from build123d import *

# Parameters (mm, degrees)
F0_W     = 125
F0_H     = 80
F0_W_2   = 121
F0_H_2   = 76
F1_DEPTH = 4
F2_W     = 121
F2_H     = 76
F3_DEPTH = 1
F4_W     = 30
F4_H     = 101.913806
F4_H_2   = 48.086194
F5_DEPTH = 10
F6_W     = 80
F6_H     = 30
F6_W_2   = 30
F6_H_2   = 10
F7_DEPTH = 5


with BuildPart() as f1:
    # F0 (on Front) → F1 (new body)
    with BuildSketch(Plane.XZ):
        Rectangle(F0_W, F0_H)
        Rectangle(F0_W_2, F0_H_2, mode=Mode.SUBTRACT)
        Rectangle(F0_W_2, F0_H_2)
    extrude(amount=F1_DEPTH)

    # F2 (on face) → F3 (cut)
    with BuildSketch(Plane.XZ.offset(4)):
        Rectangle(F2_W, F2_H)
    extrude(amount=-F3_DEPTH, mode=Mode.SUBTRACT)

    # F4 (on face) → F5 (join)
    with BuildSketch(Plane.XZ):
        with Locations((0, -88.956903)):
            Rectangle(F4_W, F4_H)
        with Locations((0, -13.956903)):
            Rectangle(F4_W, F4_H_2)
    extrude(amount=-F5_DEPTH)

    # F6 (on face) → F7 (join)
    with BuildSketch(Plane(origin=(0, 0, -139.913806), x_dir=(1, 0, 0), z_dir=(0, 0, -1))):
        with Locations((0, -5)):
            Rectangle(F6_W, F6_H)
        with Locations((0, -5)):
            Rectangle(F6_W_2, F6_H_2, mode=Mode.SUBTRACT)
    extrude(amount=-F7_DEPTH)


solid = f1.part
The listing builds one solid part. Answer for the finished solid, in the listing's coordinates (mm). A direction names the side the tool comes from. Give positions to 0.01 mm unless a question says otherwise; leave off trailing zeros. Write each loop counter-clockwise with the first axis right and the second up, starting at its lowest first coordinate (ties: lowest second). Pieces come first, ordered by that corner, then holes.
1) For a pull along Z with two mould halves and no side action, classify faces 1 (the face through (-1, 11, -134.914)), 2 (the face through (-1, 5, -139.914)), 3 (the face through (-1, 20, -137)) as pulls with the +Z half, pulls with the -Z half, needs draft (parallel to the pull), parting line crosses it, or undercut.
2) A tool of negligible diameter and unlimited length cuts with its end or side. For faces 4 (the face through (0, 10, -61)), 5 (the face through (0, -4, 39)), 6 (the face through (-1, -2, -40)), 7 (the face through (-1, -3, 1)), from which of +Z, -Z, +X, -X, +Y, -Y can it reach the whole face along a straight path? Write none if from no direction.
3) Find the intervals of material crossed by L1, parallel to Z at x = 28, y = -2.5; L2, parallel to X at y = 8.25, z = -58.5; L3, parallel to Z at x = -26, y = -5, in increasing order.
4) Section A-A (x = 32.5) is taken. Write down the section's boundary in (y, z).
5) Section D-D (y = 7.75) is taken. Write down the section's boundary in (x, z).
6) Section C-C (z = -18.5) is taken. Write down the section's boundary in (x, y), and give its area (3 significant figures).
7) Given P1, Ø4, axis at y = 6, z = -136.5, coming from the +X side; P2, Ø3, axis at y = 5.5, z = -86, coming from the -X side; P3, Ø24, axis at x = -30, z = 4.5, coming from the +Y side, each flat-ended and moving along its own axis, determine where each tip first touches the part or whether it passes through.
8) Section B-B (x = -12.5) is taken. Write down the section's boundary in (y, z).
Response:
1. face 1: undercut
1. face 2: pulls with the -Z half
1. face 3: needs draft
2. face 4: +Z, +X, -X, +Y
2. face 5: +Z, +X, -X, -Y
2. face 6: +X, -X, -Y
2. face 7: -Y
3. L1: z = -139.91 to -134.91, -40 to 40
3. L2: x = -15 to 15
3. L3: z = -139.91 to -134.91
4. outline: (-10, -139.91) - (20, -139.91) - (20, -134.91) - (-10, -134.91) - close; (-4, -40) - (0, -40) - (0, 40) - (-4, 40) - (-4, 38) - (-3, 38) - (-3, -38) - (-4, -38) - close
5. outline: (-40, -139.91) - (40, -139.91) - (40, -134.91) - (15, -134.91) - (15, 10.09) - (-15, 10.09) - (-15, -134.91) - (-40, -134.91) - close
6. outline: (-62.5, -4) - (-60.5, -4) - (-60.5, -3) - (60.5, -3) - (60.5, -4) - (62.5, -4) - (62.5, 0) - (15, 0) - (15, 10) - (-15, 10) - (-15, 0) - (-62.5, 0) - close
6. area: 679 mm2
7. P1: stops at x = 40
7. P2: stops at x = -15
7. P3: stops at y = 0
8. outline: (-10, -139.91) - (20, -139.91) - (20, -134.91) - (10, -134.91) - (10, 10.09) - (0, 10.09) - (0, 40) - (-4, 40) - (-4, 38) - (-3, 38) - (-3, -38) - (-4, -38) - (-4, -40) - (0, -40) - (0, -134.91) - (-10, -134.91) - close
